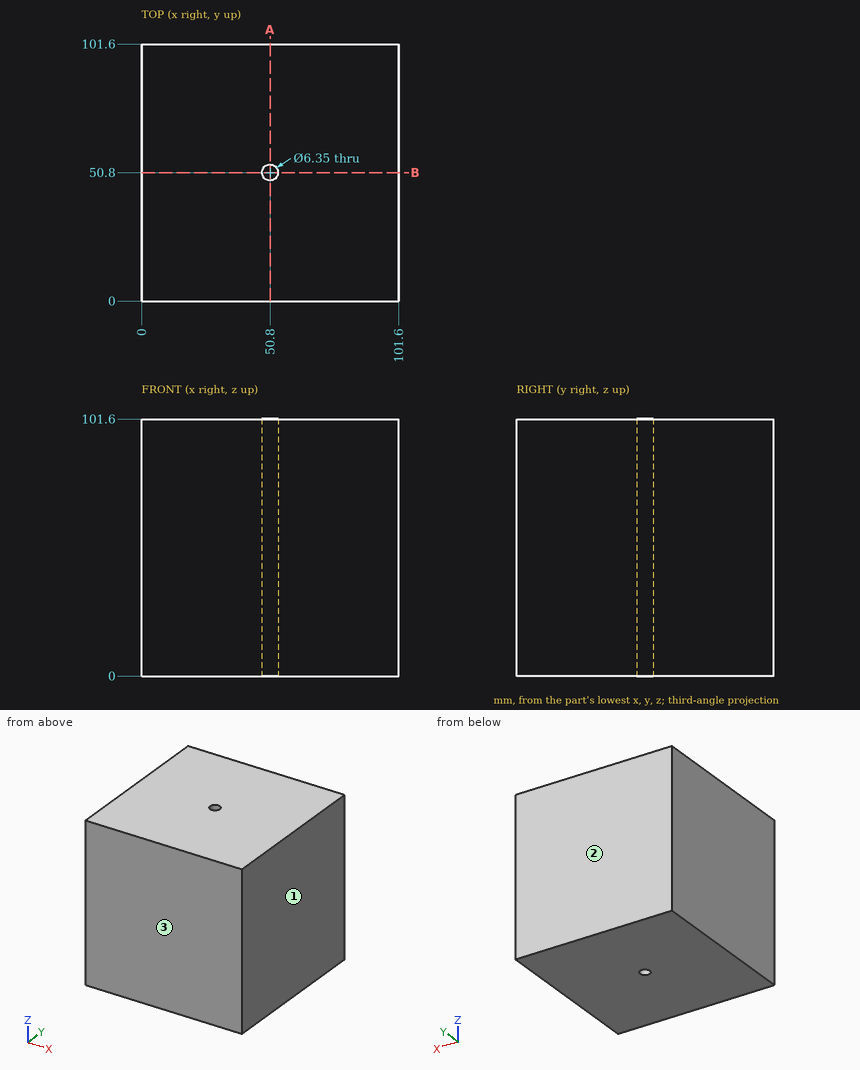
Answer from the drawing. Dimensions are ordinates in mm from the lowest x, y and z of the part. Round coordinates to 2 decimals unless told otherwise and drop trailing zeros. Write each loop counter-clockwise with the first axis right and the second up, starting at its lowest first coordinate (ties: lowest second). Pieces come first, ordered by that corner, then holes.
1. The part is cut by section A-A, the plane x = 50.8. Determine the outline of the cut face in (y, z) (3 decimals), then the cut area to 3 significant figures.
2. Straight lines are drawn through the part: L1, parallel to Y at x = 50.8, z = 44 (3 decimals); L2, parallel to X at y = 50, z = 35. For each, find the intervals that lie inside material, in ascending order.
3. Given pin 1 Ø10 at (x, y) = (50.8, 50.8) entering from +Z, flat-ended and moving along its own axis, determine where the tip first touches the part or whether it passes through.
4. Determine the mould class of the marked faces 1, 2 and 3 for opening direction Y: pulls with the +Y half, pulls with the -Y half, needs draft (parallel to the pull), parting line crosses it, or undercut.
Values:
1. outline: (0, 0) - (47.625, 0) - (47.625, 101.6) - (0, 101.6) - close; (53.975, 0) - (101.6, 0) - (101.6, 101.6) - (53.975, 101.6) - close
1. area: 9,680 mm2
2. L1: y = 0 to 47.625, 53.975 to 101.6
2. L2: x = 0 to 47.73, 53.87 to 101.6
3. pin 1: stops at z = 101.6
4. face 1: needs draft
4. face 2: pulls with the +Y half
4. face 3: pulls with the -Y half
